Autodesk Inventor part; units mm, degrees
ref_plane "YZ Plane" through (0, 0, 0) normal (1, 0, 0) x (0, 1, 0)
ref_plane "XZ Plane" through (0, 0, 0) normal (0, 1, 0) x (-1, 0, 0)
ref_plane "XY Plane" through (0, 0, 0) normal (0, 0, 1) x (1, 0, 0)
sketch "Sketch1" plane through (0, 0, 0) normal (0, 0, 1) x (1, 0, 0)
  line L0 (-12, 2.5) -> (12, 2.5)
  line L1 (12, 2.5) -> (12, -2.5)
  line L2 (12, -2.5) -> (-12, -2.5)
  line L3 (-12, -2.5) -> (-12, 2.5)
  point P0 (0, 0)
  point P1 (12, 0)
  point P2 (0, 2.5)
  dimension "d0" = 24
  dimension "d1" = 5
extrude "Extrusion1" add sketch "Sketch1" along normal blind 1
sketch "Sketch2" plane through (0, 0, 1) normal (0, 0, 1) x (1, 0, 0)
  line L0 (-9, 0) -> (9, 0) construction
  point P0 (0, 0)
  point P1 (0, 0)
  dimension "d4" = 18
hole "Hole1" at (9, 0, 1) at (-9, 0, 1) direction (0, 0, -1) diameter 2 end through all
properties part number "probe-side-large-mesh-support-plate" material "Stainless Steel"
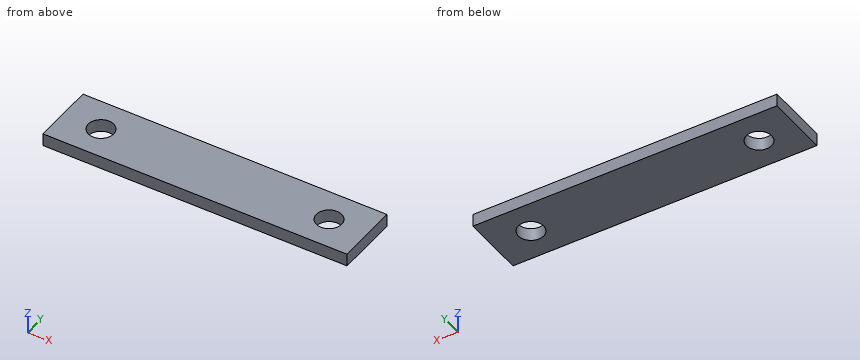
The listing builds one solid part. Answer for the finished solid, in the listing's coordinates (mm). Give positions to 0.01 mm unless a question says otherwise; leave off trailing zeros. Loops run counter-clockwise (first coordinate to the right, second up) from the corner with the lowest first, then second, coordinate; pieces in that order, holes last.
Item 1: Find the intervals of material crossed by line 1 along X through (y, z) = (0, 0.35); line 2 along Y through (x, z) = (-9, 0.55); line 3 along X through (y, z) = (-0.7, 0.7), in increasing order.
Derived:
line 1: x = -12 to -10, -8 to 8, 10 to 12
line 2: y = -2.5 to -1, 1 to 2.5
line 3: x = -12 to -9.71, -8.29 to 8.29, 9.71 to 12
Item 2: A cutting plane is placed at A-A (y = 0). Give the vertices of the cut face in (x, z).
Derived:
outline: (-12, 0) - (-10, 0) - (-10, 1) - (-12, 1) - close; (-8, 0) - (8, 0) - (8, 1) - (-8, 1) - close; (10, 0) - (12, 0) - (12, 1) - (10, 1) - close
Item 3: A cutting plane is placed at C-C (z = 0.75). Give the vertices of the cut face in (x, y), then the cut area to 3 significant figures.
Derived:
outline: (-12, -2.5) - (12, -2.5) - (12, 2.5) - (-12, 2.5) - close; hole circle Ø2 at (-9, 0); hole circle Ø2 at (9, 0)
area: 114 mm2
Item 4: A cutting plane is placed at B-B (x = 9). Give the vertices of the cut face in (y, z), then the cut area to 3 significant figures.
Derived:
outline: (-2.5, 0) - (-1, 0) - (-1, 1) - (-2.5, 1) - close; (1, 0) - (2.5, 0) - (2.5, 1) - (1, 1) - close
area: 3.00 mm2
